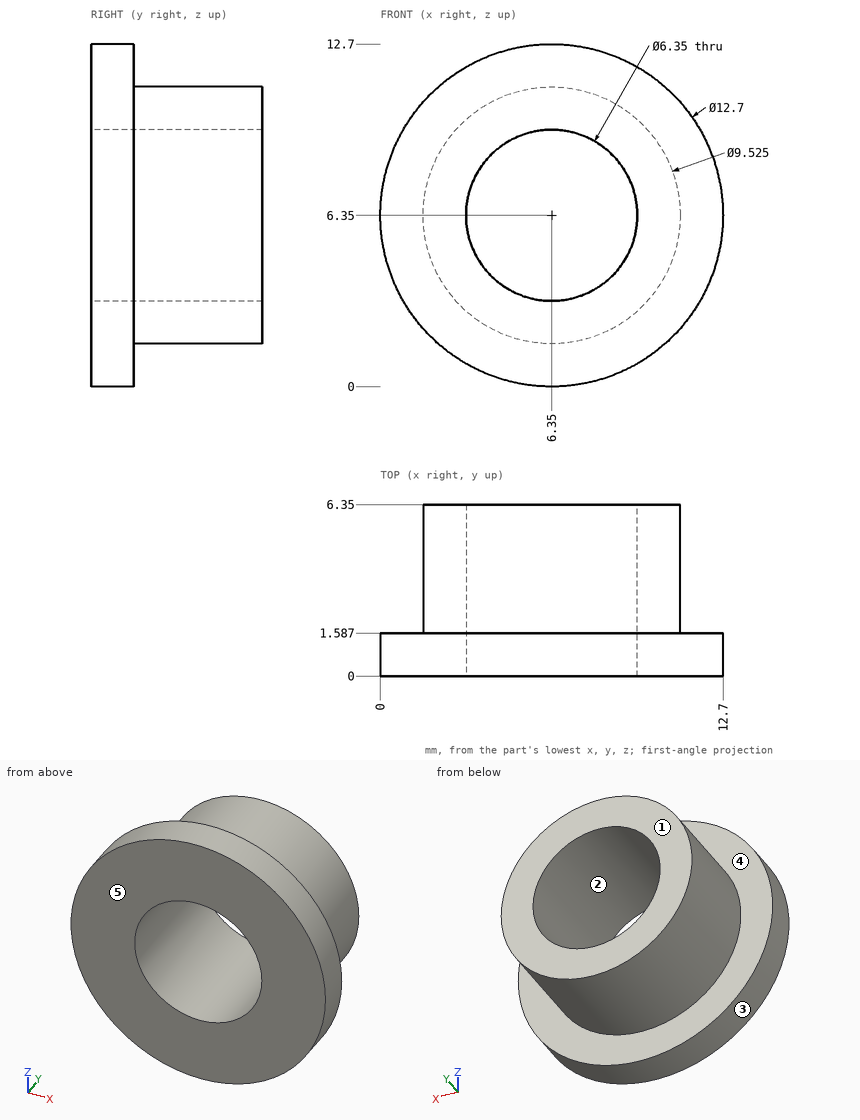
Can you work these out from the drawing? Everything is in mm from the part's minimum corner. A direction names the side the tool comes from. Coordinates: 2 decimals unless noted, no trailing zeros. Return JSON: item names as keys, results as strings.
1) Thinking about a two-plate mould opening in Z: for the marked faces 1, 2 and 3, which applies, +Z half, -Z half, draft (parallel to the pull), parting line (faces both ways), or undercut?
Results below:
{"face 1": "draft", "face 2": "undercut", "face 3": "parting line"}
2) Will these pins go through, and if not, where does the flat tip stop? pin 1 (5.5 mm diameter, centred on x = 6.35, z = 6.35, fed in from -Y); pin 2 (1 mm diameter, centred on y = 1, z = 1.5, fed in from +X) (1 decimal).
Results below:
{"pin 1": "through", "pin 2": "x = 11"}
3) For the marked faces 4 and 5, which set-ups out of +Z, -Z, +X, -X, +Y, -Y let a thin tool reach every point of the face, with its end or its side?
Results below:
{"face 4": "+Y", "face 5": "+Z, -Z, +X, -X, -Y"}
4) I need wall thicknesses on line 1 (X direction, y = 3, z = 6.35) (1 decimal); line 2 (X direction, y = 4.75, z = 5.25) (1 decimal). Which ranges of each line are inside material? Lowest first, please. Write a range as from..to.
Results below:
{"line 1": "1.6..3.2, 9.5..11.1", "line 2": "1.7..3.4, 9.3..11"}
